Print and shaded views of the part. All mm, measured from the part's lowest x, y and z. Give positions to 0.01 mm unless a question says otherwise; leave off trailing zeros. Write each loop counter-clockwise with the first axis right and the second up, starting at its lowest first coordinate (ties: lowest second). Pieces come first, ordered by that corner, then holes. Notation, with made-up numbers: (11.25, 37) -> (64.25, 37) arc R13 cw to (64.25, 51) -> close; hole circle Ø4 at (43, -34). An arc over 180 degrees is marked (long way). Put each result on its own line as item: value.
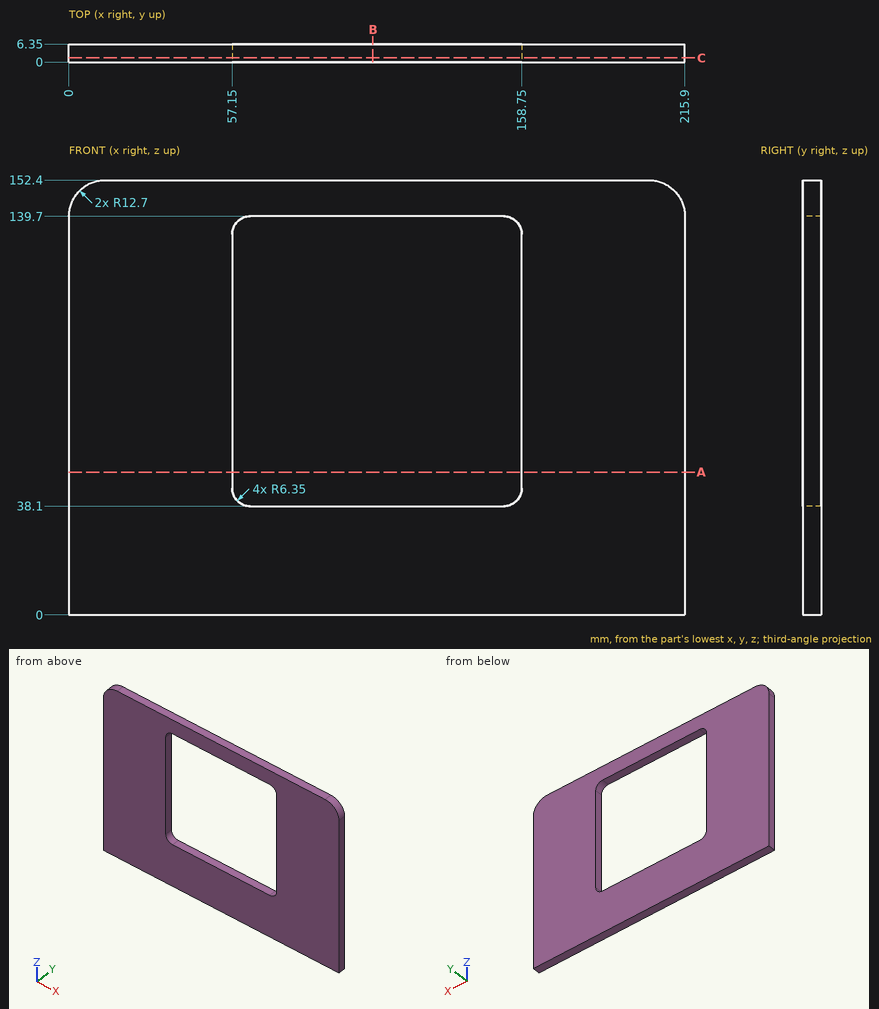
1) Pin check, flat tip, straight feed: pin 1 (1 mm diameter, centred on y = 5.5, z = 20, fed in from -X). Stop position of the tip, or through.
Filled sheet:
pin 1: x = 0
2) Slice it at B-B (x = 106.5). Write the cut outline in (y, z), plus the area to 3 significant figures.
Filled sheet:
outline: (0, 0) -> (6.35, 0) -> (6.35, 38.1) -> (0, 38.1) -> close; (0, 139.7) -> (6.35, 139.7) -> (6.35, 152.4) -> (0, 152.4) -> close
area: 323 mm2
3) Wall check: L1, parallel to X at y = 2, z = 72.5; L2, parallel to Z at x = 116, y = 5; L3, parallel to Z at x = 58.5, y = 5.5. Give the ranges that are in metal, low to high.
Filled sheet:
L1: 0 to 57.15, 158.75 to 215.9
L2: 0 to 38.1, 139.7 to 152.4
L3: 0 to 40.54, 137.26 to 152.4
4) Slice it at A-A (z = 50). Write the cut outline in (x, y).
Filled sheet:
outline: (0, 0) -> (57.15, 0) -> (57.15, 6.35) -> (0, 6.35) -> close; (158.75, 0) -> (215.9, 0) -> (215.9, 6.35) -> (158.75, 6.35) -> close
5) Slice it at C-C (y = 1.5). Write the cut outline in (x, z).
Filled sheet:
outline: (0, 0) -> (215.9, 0) -> (215.9, 139.7) arc R12.7 ccw to (203.2, 152.4) -> (12.7, 152.4) arc R12.7 ccw to (0, 139.7) -> close; hole (57.15, 44.45) arc R6.35 ccw to (63.5, 38.1) -> (152.4, 38.1) arc R6.35 ccw to (158.75, 44.45) -> (158.75, 133.35) arc R6.35 ccw to (152.4, 139.7) -> (63.5, 139.7) arc R6.35 ccw to (57.15, 133.35) -> close
